Input: part model. Units: mm. Frame: model coordinates. A direction names the side the tool comes from. Coordinates: 2 decimals unless noted, no trailing zeros. Write each loop counter-clockwise with the first axis right and the second up, starting at its lowest first coordinate (ties: lowest second). Pieces come first, ordered by that corner, then holes. Notation, with made-up numbers: (79.25, -32) - (108.25, -32) arc R23 cw to (108.25, -18) - close; hole circle Ø4 at (18, 48). An arc over 180 degrees is marked (long way). Put each result on its own line as item: value. Start each with the question number.
1. Cut plane B-B, the plane y = 3.75. Return loops of the section in (x, z) (3 decimals), and give its area (3 significant figures).
2. Pull-direction query (X, two-part tool) for faces 1 (the flat face through (2.2, 0, 0)), 2 (the cylindrical face through (-1.147, 1.735, 2.767)), 3 (the flat face through (0, 2.75, 2.3)); classes: released by +X, released by -X, zero draft, split by the parting line, or undercut.
3. Pin query (flat end, axial travel): pin 1 (2.5 mm diameter, centred on x = 0, z = 0, fed in from -Y); pin 2 (0.6 mm diameter, centred on y = 1.5, z = -2.5, fed in from -X); pin 3 (1.3 mm diameter, centred on y = 1, z = -2.5, fed in from +X); pin 4 (1 mm diameter, centred on y = 1.5, z = -1, fed in from -X). Return the tip coordinate at first contact, or that it passes through.
4. Access query for faces 4 (the flat face through (0.84, 1, -2)), 5 (the flat face through (-2.1, 0, 0)). Directions: +Z, -Z, +X, -X, +Y, -Y. A direction counts if a zero-diameter tool reaches every point of the face in a straight line with its end or side. Return the directions, or none.
5. Line query: line 1 (X direction, y = 3, z = 0) (3 decimals); line 2 (Z direction, x = -0.1, y = 4.5); line 3 (X direction, y = 5.5, z = -0.8). Output: solid intervals per line, ascending.
6. Cut plane A-A, the plane y = 0.5. Return loops of the section in (x, z) (3 decimals), and give its area (3 significant figures).
from build123d import *
from build123d.topology import SkipClean

# Parameters (mm, degrees)
SKETCH1_R               = 2.995
BOSS_EXTRUDE1_DEPTH     = 3.52
SKETCH2_R               = 2.425
SKETCH2_R_2             = 1.975
BOSS_EXTRUDE2_DEPTH     = 2.53
THREAD1_PITCH           = 0.8
SKETCH6_R               = 3.05
SKETCH6_R_2             = 2.425
CUT_EXTRUDE1_DEPTH      = 1.1
SKETCH7_R               = 1.875
CUT_EXTRUDE2_DEPTH      = 3
CUT_EXTRUDE4_DEPTH      = 8.385434789
CUT_EXTRUDE4_DEPTH_BACK = 8.385434789
SKETCH9_W               = 1.68
SKETCH9_H               = 2.75
CUT_EXTRUDE6_START      = -3.18
SKETCH10_R              = 1.975
CUT_EXTRUDE6_DEPTH      = 3.18


with BuildPart() as part:
    # Sketch1 → Boss-Extrude1 (new body)
    with BuildSketch(Plane(origin=(0, 0, 0), x_dir=(1, 0, 0), z_dir=(0, 1, 0))):
        with Locations(Location((0, 0, 0), (0, 0, 270))):
            Circle(SKETCH1_R)
    extrude(amount=BOSS_EXTRUDE1_DEPTH)

    # Sketch2 → Boss-Extrude2 (add)
    with BuildSketch(Plane(origin=(0, 3.52, 0), x_dir=(1, 0, 0), z_dir=(0, 1, 0))):
        with Locations(Location((0, 0, 0), (0, 0, 270))):
            Circle(SKETCH2_R)
        with Locations(Location((0, 0, 0), (0, 0, 270))):
            Circle(SKETCH2_R_2, mode=Mode.SUBTRACT)
    extrude(amount=BOSS_EXTRUDE2_DEPTH)

    # Thread1: the profile of Thread Profile1 profile screwed along a right-hand helix of 1.875 turns, 8 arcs to a turn; built about Z, then put on its axis
    thread1_z = Axis((0, 0, 0), (0, 0, 1))
    thread1_corners = [(2.4247, 0, -0.000173205), (2.4247, 0, 0.700173203), (2.8580127, 0, 0.449999999), (2.8580127, 0, 0.249999999)]
    with BuildLine(mode=Mode.PRIVATE) as thread1_profile:
        Line(thread1_corners[0], thread1_corners[1])
        Line(thread1_corners[1], thread1_corners[2])
        Line(thread1_corners[2], thread1_corners[3])
        Line(thread1_corners[3], thread1_corners[0])
    thread1_cap = Face(thread1_profile.wire())
    thread1_turn_angles = [0, 22.5, 45, 67.5, 90, 112.5, 135, 157.5, 180, 202.5, 225, 247.5, 270, 292.5, 315, 337.5, 360]
    thread1_turn_weights = [1, 0.9238795325112867, 1, 0.9238795325112867, 1, 0.9238795325112867, 1, 0.9238795325112867, 1, 0.9238795325112867, 1, 0.9238795325112867, 1, 0.9238795325112867, 1, 0.9238795325112867, 1]
    thread1_turn_rails = [Edge.make_bspline([Vector(p[0], p[1], 0).rotate(thread1_z, thread1_turn_angles[k]) / thread1_turn_weights[k] + Vector(0, 0, p[2] + THREAD1_PITCH * thread1_turn_angles[k] / 360) for k in range(17)], [0, 0, 0, 1, 1, 2, 2, 3, 3, 4, 4, 5, 5, 6, 6, 7, 7, 8, 8, 8], 2, thread1_turn_weights) for p in thread1_corners]
    thread1_turn_sides = [Face.make_surface_from_curves(thread1_turn_rails[p[0]], thread1_turn_rails[p[1]]) for p in [(0, 1), (1, 2), (2, 3), (3, 0)]]
    thread1_last_angles = [360, 382.5, 405, 427.5, 450, 472.5, 495, 517.5, 540, 562.5, 585, 607.5, 630, 652.5, 675]
    thread1_last_weights = [1, 0.9238795325112867, 1, 0.9238795325112867, 1, 0.9238795325112867, 1, 0.9238795325112867, 1, 0.9238795325112867, 1, 0.9238795325112867, 1, 0.9238795325112867, 1]
    thread1_last_rails = [Edge.make_bspline([Vector(p[0], p[1], 0).rotate(thread1_z, thread1_last_angles[k]) / thread1_last_weights[k] + Vector(0, 0, p[2] + THREAD1_PITCH * thread1_last_angles[k] / 360) for k in range(15)], [0, 0, 0, 1, 1, 2, 2, 3, 3, 4, 4, 5, 5, 6, 6, 7, 7, 7], 2, thread1_last_weights) for p in thread1_corners]
    thread1_last_sides = [Face.make_surface_from_curves(thread1_last_rails[p[0]], thread1_last_rails[p[1]]) for p in [(0, 1), (1, 2), (2, 3), (3, 0)]]
    thread1 = Plane(origin=(0, 6.05, 0), x_dir=(-1, 0, 0), z_dir=(0, -1, 0)) * Solid(Shell([*thread1_turn_sides, *thread1_last_sides, thread1_cap, thread1_cap.rotate(thread1_z, 675).moved(Location((0, 0, THREAD1_PITCH * 675 / 360)))]))
    add(thread1)

    # Sketch6 → Cut-Extrude1 (cut)
    with BuildSketch(Plane(origin=(0, 3.52, 0), x_dir=(1, 0, 0), z_dir=(0, 1, 0))):
        Circle(SKETCH6_R)
        with Locations(Location((0, 0, 0), (0, 0, 180))):
            Circle(SKETCH6_R_2, mode=Mode.SUBTRACT)
    extrude(amount=CUT_EXTRUDE1_DEPTH, mode=Mode.SUBTRACT)

    # Sketch7 → Cut-Extrude2 (cut)
    with BuildSketch(Plane.XZ):
        with Locations(Location((0, 0, 0), (0, 0, 270))):
            Circle(SKETCH7_R)
    extrude(amount=-CUT_EXTRUDE2_DEPTH, mode=Mode.SUBTRACT)

    # Sketch9 → Cut-Extrude4 (cut, two sides: drawn at the far end of the back side and taken through both)
    with BuildSketch(Plane.XY.offset(-CUT_EXTRUDE4_DEPTH_BACK)):
        with Locations((0, 1.375)):
            Rectangle(SKETCH9_W, SKETCH9_H)
    extrude(amount=CUT_EXTRUDE4_DEPTH + CUT_EXTRUDE4_DEPTH_BACK, mode=Mode.SUBTRACT)

    # Sketch10 → Cut-Extrude6 (cut)
    with SkipClean():  # the faces are left unmerged after this step: merging them gives an invalid solid
        with BuildSketch(Plane(origin=(0, 6.05, 0), x_dir=(1, 0, 0), z_dir=(0, 1, 0)).offset(CUT_EXTRUDE6_START)):
            with Locations(Location((0, 0, 0), (0, 0, 270))):
                Circle(SKETCH10_R)
        extrude(amount=CUT_EXTRUDE6_DEPTH, mode=Mode.SUBTRACT)


solid = part.part
Report:
1. outline: circle Ø4.85 at (0, 0); hole circle Ø3.95 at (0, 0)
1. area: 6.22 mm^2
2. face 1: zero draft
2. face 2: split by the parting line
2. face 3: undercut
3. pin 1: passes through
3. pin 2: stops at x = -2.03
3. pin 3: stops at x = 2.36
3. pin 4: stops at x = -2.95
4. face 4: +Z, -Z, -Y
4. face 5: +Z, -Z, +X, -X, -Y
5. line 1: x = -2.995 to -1.975, 1.975 to 2.995
5. line 2: z = -2.42 to -1.97, 1.97 to 2.42
5. line 3: x = -2.63 to -1.81, 1.81 to 2.63
6. outline: (-0.84, -2.875) - (-0.84, -1.676) arc R1.875 cw to (-0.84, 1.676) - (-0.84, 2.875) arc R2.995 ccw to start; (0.84, -2.875) arc R2.995 ccw to (0.84, 2.875) - (0.84, 1.676) arc R1.875 cw to (0.84, -1.676) - close
6. area: 13.3 mm^2
